```python
from build123d import *

# Parameters (mm, degrees)
SKETCH3_R = 0.3937


with BuildPart() as part:
    # Sweep3: sweep along a curve in space
    with BuildLine() as sweep3_path:
        Line((-15.494, 0.5969, -1.778), (-15.494, -14.478, -1.778))
        ThreePointArc((-14.3129, 1.778, -1.778), (-15.148063819, 1.432063819, -1.778), (-15.494, 0.5969, -1.778))
        Line((6.1849, 1.778, -1.778), (-14.3129, 1.778, -1.778))
        ThreePointArc((7.366, 1.778, -2.9591), (7.020063819, 1.778, -2.123936181), (6.1849, 1.778, -1.778))
        Line((7.366, 1.778, -2.9591), (7.366, 1.778, -4.6863))
        ThreePointArc((8.752195863, 1.778, -5.849456437), (7.787903554, 1.778, -5.591075092), (7.366, 1.778, -4.6863))
        Line((8.752195863, 1.778, -5.849456437), (26.289, 1.778, -2.757244712))
    # Sketch3 → Sweep3 (sweep)
    with BuildSketch(Plane(origin=(-15.494, -14.478, -1.778), x_dir=(1, 0, 0), z_dir=(0, -1, 0))):
        Circle(SKETCH3_R)
    sweep(path=sweep3_path.line)


solid = part.part
```
For this review, take the finished solid that the model builds, in its own axes (mm). Give positions to 0.01 mm unless a question says otherwise; leave off trailing zeros. Order: outer loops, then holes, each group sorted by start corner. A loop starts at its lowest first (then second) coordinate and runs counter-clockwise, first axis right, second up.
1) Insertion check: pin 1 (2 mm diameter, centred on x = 8, z = -4.5, fed in from -Y); pin 2 (2 mm diameter, centred on y = -10, z = -5, fed in from +X). Each pin has a flat end and moves straight along its axis. Give the tip position at first contact, or say it passes through.
2) Take a section at A-A (y = -3.25). Give the boundary of the cut face in (x, z), then the cut area to 3 significant figures.
3) Take a section at B-B (x = -3.5). Give the boundary of the cut face in (y, z), then the cut area to 3 significant figures.
4) Wall thickness on line 1 (Y direction, x = -7.5, z = -1.7); line 2 (X direction, y = -9.25, z = -1.8); line 3 (X direction, y = -9.5, z = -1.6): over which ranges is each line inside the solid? List them lowest first.
Derived:
1. pin 1: stops at y = 1.38
1. pin 2: passes through
2. outline: circle Ø0.79 at (-15.49, -1.78)
2. area: 0.487 mm2
3. outline: circle Ø0.79 at (1.78, -1.78)
3. area: 0.487 mm2
4. line 1: y = 1.39 to 2.16
4. line 2: x = -15.89 to -15.1
4. line 3: x = -15.85 to -15.14
